```python
from build123d import *

# Parameters (mm, degrees)
SKETCH3_W                       = 80
SKETCH3_H                       = 80
SKETCH3_W_2                     = 60
SKETCH3_H_2                     = 60
BOSS_EXTRUDE2_DEPTH             = 1600
SKETCH7_W                       = 60
SKETCH7_H                       = 60
BOSS_EXTRUDE3_DEPTH             = 5
BOSS_EXTRUDE4_REACH             = 1610.361
SKETCH8_W                       = 205
SKETCH8_H                       = 5
BOSS_EXTRUDE4_DIRECTION_2_REACH = 1610.361
CUT_EXTRUDE1_DEPTH              = 5
CUT_EXTRUDE2_REACH              = 1612.59
FILLET1_R                       = 5
FILLET1_OF_MIRROR1_R            = 5
FILLET1_OF_MIRROR2_R            = 5


with BuildPart() as part:
    # Sketch3 → Boss-Extrude2 (new body)
    with BuildSketch(Plane(origin=(0, 0, 0), x_dir=(0, 0, -1), z_dir=(1, 0, 0))):
        with Locations((40, 40)):
            Rectangle(SKETCH3_W, SKETCH3_H)
        with Locations((40, 40)):
            Rectangle(SKETCH3_W_2, SKETCH3_H_2, mode=Mode.SUBTRACT)
    extrude(amount=BOSS_EXTRUDE2_DEPTH)

    # Sketch7 → Boss-Extrude3 (add)
    with BuildSketch(Plane(origin=(1530, 0, 0), x_dir=(0, 0, -1), z_dir=(1, 0, 0))):
        Polygon((-60, 85), (140, 85), (140, 5), (90, -35), (-10, -35), (-60, 5), align=None)
        with Locations((40, 40)):
            Rectangle(SKETCH7_W, SKETCH7_H, mode=Mode.SUBTRACT)
    boss_extrude3 = extrude(amount=BOSS_EXTRUDE3_DEPTH)

    # Boss-Extrude4: up to this face of the body (flat: up to its plane)
    boss_extrude4_end = Plane(part.part.faces().sort_by_distance((1532.5, 45, -140))[0])
    # Sketch8 → Boss-Extrude4 (add, up to the picked face)
    with BuildSketch(Plane(origin=(0, 0, -80), x_dir=(-1, 0, 0), z_dir=(0, 0, -1)), mode=Mode.PRIVATE) as boss_extrude4_sk1:
        with Locations((-1432.5, 82.5)):
            Rectangle(SKETCH8_W, SKETCH8_H)
    boss_extrude4_tool1 = split(extrude(boss_extrude4_sk1.sketch, amount=BOSS_EXTRUDE4_REACH, mode=Mode.PRIVATE), bisect_by=boss_extrude4_end, keep=Keep.BOTH, mode=Mode.PRIVATE)
    boss_extrude4 = boss_extrude4_tool1.solids().sort_by(Axis((1432.5, 82.5, -80), (0, 0, -1)))[0]
    add(boss_extrude4)

    # Boss-Extrude4 direction 2: up to this face of the body (flat: up to its plane)
    boss_extrude4_direction_2_end = Plane(part.part.faces().sort_by_distance((1532.5, 45, 60))[0])
    # Sketch8 → Boss-Extrude4 direction 2 (add, up to the picked face)
    with BuildSketch(Plane(origin=(0, 0, -80), x_dir=(-1, 0, 0), z_dir=(0, 0, -1)), mode=Mode.PRIVATE) as boss_extrude4_direction_2_sk1:
        with Locations((-1432.5, 82.5)):
            Rectangle(SKETCH8_W, SKETCH8_H)
    boss_extrude4_direction_2_tool1 = split(extrude(boss_extrude4_direction_2_sk1.sketch, amount=-BOSS_EXTRUDE4_DIRECTION_2_REACH, mode=Mode.PRIVATE), bisect_by=boss_extrude4_direction_2_end, keep=Keep.BOTH, mode=Mode.PRIVATE)
    boss_extrude4_direction_2 = boss_extrude4_direction_2_tool1.solids().sort_by(Axis((1432.5, 82.5, -80), (0, 0, 1)))[0]
    add(boss_extrude4_direction_2)

    # Sketch9 → Cut-Extrude1 (cut)
    with BuildSketch(Plane(origin=(0, 85, 0), x_dir=(1, 0, 0), z_dir=(0, 1, 0))):
        with BuildLine():
            Line((1330, 80), (1335.801257358, 71.298113962))
            ThreePointArc((1335.801257358, 71.298113962), (1338.927300662, 64.675212774), (1340, 57.430609057))
            Line((1340, 57.430609057), (1340, 22.569390943))
            ThreePointArc((1340, 22.569390943), (1338.927300662, 15.324787226), (1335.801257358, 8.701886038))
            Line((1335.801257358, 8.701886038), (1330, 0))
            Line((1330, 0), (1330, 80))
        make_face()
    cut_extrude1 = extrude(amount=-CUT_EXTRUDE1_DEPTH, mode=Mode.SUBTRACT)

    # Sketch10 → Cut-Extrude2 (cut, up to next)
    with BuildSketch(Plane(origin=(0, 85, 0), x_dir=(1, 0, 0), z_dir=(0, 1, 0)), mode=Mode.PRIVATE) as cut_extrude2_sk1:
        with BuildLine():
            Line((1342.5, 126), (1522.5, 126))
            ThreePointArc((1522.5, 126), (1528.5, 120), (1522.5, 114))
            Line((1522.5, 114), (1342.5, 114))
            ThreePointArc((1342.5, 114), (1336.5, 120), (1342.5, 126))
        make_face()
    cut_extrude2_tool1 = extrude(cut_extrude2_sk1.sketch, amount=-CUT_EXTRUDE2_REACH, mode=Mode.PRIVATE) & part.part
    # Sketch10 → Cut-Extrude2 (cut, up to next)
    with BuildSketch(Plane(origin=(0, 85, 0), x_dir=(1, 0, 0), z_dir=(0, 1, 0)), mode=Mode.PRIVATE) as cut_extrude2_sk2:
        with BuildLine():
            Line((1342.5, -34), (1522.5, -34))
            ThreePointArc((1522.5, -34), (1528.5, -40), (1522.5, -46))
            Line((1522.5, -46), (1342.5, -46))
            ThreePointArc((1342.5, -46), (1336.5, -40), (1342.5, -34))
        make_face()
    cut_extrude2_tool2 = extrude(cut_extrude2_sk2.sketch, amount=-CUT_EXTRUDE2_REACH, mode=Mode.PRIVATE) & part.part
    cut_extrude2_1 = cut_extrude2_tool1.solids().sort_by_distance((1432.5, 85, -120))[0]
    add(cut_extrude2_1, mode=Mode.SUBTRACT)
    cut_extrude2_2 = cut_extrude2_tool2.solids().sort_by_distance((1432.5, 85, 40))[0]
    add(cut_extrude2_2, mode=Mode.SUBTRACT)
    cut_extrude2 = cut_extrude2_1 + cut_extrude2_2  # Cut-Extrude2 as one shape, for the pattern or mirror that repeats it

    # Fillet1
    fillet1_edges = [part.edges().sort_by_distance(p)[0] for p in [
        (1535, 85, -40),
    ]]
    fillet(fillet1_edges, radius=FILLET1_R - 0.0001)  # a hair under: the kernel refuses the full size

    # Mirror1: Boss-Extrude3 across plane
    add(boss_extrude3.mirror(Plane(origin=(800, 0, 0), x_dir=(0, 0, 1), z_dir=(1, 0, 0))))

    # Fillet1 of Mirror1
    fillet1_of_mirror1_edges = [part.edges().sort_by_distance(p)[0] for p in [
        (65, 85, -40),
    ]]
    fillet(fillet1_of_mirror1_edges, radius=FILLET1_OF_MIRROR1_R - 0.0001)  # a hair under: the kernel refuses the full size

    # Mirror2: Boss-Extrude3, Boss-Extrude4, Boss-Extrude4 direction 2, Cut-Extrude1, Cut-Extrude2 across plane
    add(boss_extrude3.mirror(Plane(origin=(800, 0, 0), x_dir=(0, 0, 1), z_dir=(1, 0, 0))))
    add(boss_extrude4.mirror(Plane(origin=(800, 0, 0), x_dir=(0, 0, 1), z_dir=(1, 0, 0))))
    add(boss_extrude4_direction_2.mirror(Plane(origin=(800, 0, 0), x_dir=(0, 0, 1), z_dir=(1, 0, 0))))
    add(cut_extrude1.mirror(Plane(origin=(800, 0, 0), x_dir=(0, 0, 1), z_dir=(1, 0, 0))), mode=Mode.SUBTRACT)
    add(cut_extrude2.mirror(Plane(origin=(800, 0, 0), x_dir=(0, 0, 1), z_dir=(1, 0, 0))), mode=Mode.SUBTRACT)

    # Fillet1 of Mirror2
    fillet1_of_mirror2_edges = [part.edges().sort_by_distance(p)[0] for p in [
        (65, 85, -40),
    ]]
    fillet(fillet1_of_mirror2_edges, radius=FILLET1_OF_MIRROR2_R - 0.0001)  # a hair under: the kernel refuses the full size


solid = part.part
```
Could you check a few things on this model? Use its own coordinates, in mm. A direction names the side the tool comes from. Give positions to 0.01 mm unless a question says otherwise; leave off trailing zeros. Write each loop counter-clockwise with the first axis right and the second up, starting at its lowest first coordinate (ties: lowest second). Pieces come first, ordered by that corner, then holes. Notation, with made-up numbers: (-22.75, 24.25) - (13.25, 24.25) arc R33 ccw to (13.25, 55.25) - close; hole circle Ø1 at (4.5, 24). An arc over 180 degrees is marked (long way). One line per item, written item: value. Start each with the question number.
Item 1: Imagine slicing it at B-B, the plane x = 560.5. List the corners of the cut face in (y, z) for me, and give its area (3 significant figures).
Item 2: If we mould it in two halves opening along X, with no side actions, what happens to faces 4 (the face through (169, 80, 30)), 5 (the face through (32, 39, 0)), 6 (the face through (1530, -2, -41))? For each: +X half, -X half, draft (parallel to the pull), parting line (faces both ways), or undercut.
Item 3: Please list where these lines run through material, in increasing order: line 1 (Y direction, x = 171, z = -28); line 2 (Z direction, x = 1047, y = 40.5); line 3 (X direction, y = 8, z = 44). Write a range as from..to.
Item 4: Imagine slicing it at A-A, the plane y = 49. List the corners of the cut face in (x, z) for me.
Item 5: Which directions (+Z, -Z, +X, -X, +Y, -Y) give clear straight access to the entire face, cutting with the end or side of a thin tool? Please do faces 1 (the face through (1431, 80, 30)), 2 (the face through (789, 70, -40)), 3 (the face through (790, 0, -39)).
Item 6: I'm going to push flat-ended pins straight in: pin 1 (10 mm diameter, centred on x = 299, y = 26.5, fed in from -Z); pin 2 (1.5 mm diameter, centred on y = 83.5, z = 34.5, fed in from +X); pin 3 (5 mm diameter, centred on x = 864, z = -82, fed in from -Y). Where does each tip first touch, or does it pass through?
Geometry says:
1. outline: (0, -80) - (80, -80) - (80, 0) - (0, 0) - close; hole (10, -70) - (70, -70) - (70, -10) - (10, -10) - close
1. area: 2,800 mm^2
2. face 4: undercut
2. face 5: draft
2. face 6: undercut
3. line 1: 0..10, 70..85
3. line 2: -80..-70, -10..0
3. line 3: 65..70, 1530..1535
4. outline: (0, -80) - (65, -80) - (65, -140) - (70, -140) - (70, -80) - (1530, -80) - (1530, -140) - (1535, -140) - (1535, -80) - (1600, -80) - (1600, -70) - (0, -70) - close; (0, -10) - (1600, -10) - (1600, 0) - (1535, 0) - (1535, 60) - (1530, 60) - (1530, 0) - (70, 0) - (70, 60) - (65, 60) - (65, 0) - (0, 0) - close
5. face 1: +Z, -Y
5. face 2: +X, -X
5. face 3: +Z, -Z, -Y
6. pin 1: z = -80
6. pin 2: x = 1534.18
6. pin 3: y = 0
